Geometry: final body of the model. Coordinates: model frame, mm. A direction names the side the tool comes from. Round coordinates to 2 decimals unless told otherwise and drop trailing zeros. Write each loop counter-clockwise with the first axis right and the second up, starting at its lowest first coordinate (ties: lowest second). Pieces come first, ordered by that corner, then holes. Notation, with made-up numbers: (20, 83) -> (71, 83) arc R14 cw to (71, 101) -> close; hole circle Ø11 at (65.25, 53.5). An arc over 180 degrees is marked (long way). One line per item, written item: value. Start each with the question number.
from build123d import *

# Parameters (mm, degrees)
F0_R     = 0.508
F1_DEPTH = 1.016


with BuildPart() as f1:
    # F0 (on Front) → F1 (new body)
    with BuildSketch(Plane.XZ):
        with BuildLine():
            Line((0, 3.175), (0, 0.762))
            ThreePointArc((0, 0.762), (0.223185, 0.223185), (0.762, 0))
            Line((0.762, 0), (5.588, 0))
            ThreePointArc((5.588, 0), (6.126815, 0.223185), (6.35, 0.762))
            Line((6.35, 0.762), (6.35, 3.175))
            Line((6.35, 3.175), (6.672437, 3.175))
            ThreePointArc((6.672437, 3.175), (7.002393, 3.3655), (7.002393, 3.7465))
            Line((7.002393, 3.7465), (0.21997, 15.494))
            ThreePointArc((0.21997, 15.494), (-0.058941, 15.772911), (-0.439941, 15.875))
            Line((-0.439941, 15.875), (-2.573652, 15.875))
            ThreePointArc((-2.573652, 15.875), (-3.651282, 15.428631), (-4.097652, 14.351))
            Line((-4.097652, 14.351), (-4.097652, 5.715))
            ThreePointArc((-4.097652, 5.715), (-3.353703, 3.918949), (-1.557652, 3.175))
            Line((-1.557652, 3.175), (0, 3.175))
        make_face()
        with Locations((-2.048826, 5.5626)):
            Circle(F0_R, mode=Mode.SUBTRACT)
        with Locations((-2.048826, 9.525)):
            Circle(F0_R, mode=Mode.SUBTRACT)
        with Locations((-2.048826, 13.4874)):
            Circle(F0_R, mode=Mode.SUBTRACT)
    extrude(amount=F1_DEPTH)


solid = f1.part
(1) Section query A-A (y = -0.7). Count the separate pieces of the cut face and the enclosed holes in it, and give its area (3 significant figures).
(2) Set-up query: faces 4 (the face through (6.35, -0.5, 2)), 5 (the face through (-1.78, -0.5, 13.92)), 6 (the face through (0, -0.5, 2)). Return all of +Z, -Z, +X, -X, +Y, -Y with unobstructed straight access to the full face (end or side cutting, diameter ignored); none if empty.
(3) Pull-direction query (X, two-part tool) for faces 1 (the face through (-1.776, -0.501, 9.953)), 2 (the face through (-1.5, -0.5, 15.875)), 3 (the face through (-3.64, -0.5, 15.44)); classes: pulls with the +X half, pulls with the -X half, needs draft (parallel to the pull), parting line crosses it, or undercut.
(4) Line query: probe 1 along Z at (x, y) = (-0.5, -0.6) (3 decimals); probe 2 along X at (y, z) = (-0.4, 3); probe 3 along X at (y, z) = (-0.6, 5.5). Output: solid intervals per line, ascending.
(5) Pin query (flat end, axial travel): pin 1 (0.5 mm diameter, centred on y = -0.5, z = 2, fed in from +X). Return the tip coordinate at first contact, or that it passes through.
(6) Section query B-B (x = -1.75). Output: boundary loops of the cut face in (y, z) (3 decimals), and give its area (3 significant figures).
(7) Section query D-D (x = 3.5). Output: boundary loops of the cut face in (y, z), and give its area (3 significant figures).
(8) Section query C-C (z = 2.5). Output: boundary loops of the cut face in (x, y), and give its area (3 significant figures).
Results list:
1. separate pieces: 1
1. enclosed holes: 3
1. area: 114 mm^2
2. face 4: -Z, +X, +Y, -Y
2. face 5: +Y, -Y
2. face 6: -Z, -X, +Y, -Y
3. face 1: undercut
3. face 2: needs draft
3. face 3: pulls with the -X half
4. probe 1: z = 3.175 to 15.875
4. probe 2: x = 0 to 6.35
4. probe 3: x = -4.09 to -2.55, -1.54 to 5.99
5. pin 1: stops at x = 6.35
6. outline: (-1.016, 3.182) -> (0, 3.182) -> (0, 5.152) -> (-1.016, 5.152) -> close; (-1.016, 5.973) -> (0, 5.973) -> (0, 9.114) -> (-1.016, 9.114) -> close; (-1.016, 9.936) -> (0, 9.936) -> (0, 13.077) -> (-1.016, 13.077) -> close; (-1.016, 13.898) -> (0, 13.898) -> (0, 15.875) -> (-1.016, 15.875) -> close
6. area: 10.4 mm^2
7. outline: (-1.02, 0) -> (0, 0) -> (0, 9.81) -> (-1.02, 9.81) -> close
7. area: 9.97 mm^2
8. outline: (0, -1.02) -> (6.35, -1.02) -> (6.35, 0) -> (0, 0) -> close
8. area: 6.45 mm^2
